Autodesk Inventor part; units mm, degrees
ref_plane "YZ Plane" through (0, 0, 0) normal (1, 0, 0) x (0, 1, 0)
ref_plane "XZ Plane" through (0, 0, 0) normal (0, 1, 0) x (-1, 0, 0)
ref_plane "XY Plane" through (0, 0, 0) normal (0, 0, 1) x (1, 0, 0)
sketch "Skizze2" plane through (0, 0, 0) normal (0, 1, 0) x (-1, 0, 0)
  line L0 (150, 125) -> (-150, 125)
  line L1 (-150, 125) -> (-150, -125)
  line L2 (-150, -125) -> (150, -125)
  line L3 (150, -125) -> (150, 125)
  point P0 (0, 0)
  dimension "d0" = 300
  dimension "d1" = 250
  dimension "d6" = 125
  dimension "d7" = 150
extrude "Extrusion1" add sketch "Skizze2" along normal blind 15
sketch "Skizze3" plane through (0, 15, 0) normal (0, 1, 0) x (1, 0, 0)
  circle A0 centre (0, -70.5) radius 3.25
  circle A1 centre (0, 70.5) radius 3.25
  point P0 (0, 0)
  dimension "d8" = 6.5
  dimension "d9" = 6.5
  dimension "d16" = 70.5
  dimension "d17" = 70.5
extrude "Extrusion2" cut sketch "Skizze3" against normal blind 15
sketch "Skizze4" plane through (0, 0, 0) normal (0, -1, 0) x (1, 0, 0)
  circle A0 centre (0, 70.5) radius 6.5
  circle A1 centre (0, -70.5) radius 6.5
  point P0 (0, 0)
  dimension "d12" = 13
  dimension "d13" = 13
  dimension "d18" = 70.5
  dimension "d19" = 70.5
extrude "Extrusion3" cut sketch "Skizze4" against normal blind 7
chamfer "Fase1" distance 2 angle 45 4 edges at (0, 15, 125) (150, 15, 0) (0, 15, -125) (-150, 15, 0)
sketch "Skizze5" plane through (0, 15, 0) normal (0, 1, 0) x (1, 0, 0)
  circle A0 centre (142.5, -42.5) radius 2.5
  circle A1 centre (97.5, -42.5) radius 2.5
  circle A2 centre (-142.5, 42.5) radius 2.5
  circle A3 centre (-97.5, 42.5) radius 2.5
  point P0 (0, 0)
  dimension "d23" = 5
  dimension "d24" = 5
  dimension "d25" = 5
  dimension "d26" = 5
extrude "Extrusion4" cut sketch "Skizze5" against normal blind 20
thread "Gewinde1"
thread "Gewinde2"
thread "Gewinde3"
thread "Gewinde4"
properties part number "Bodenplatte"
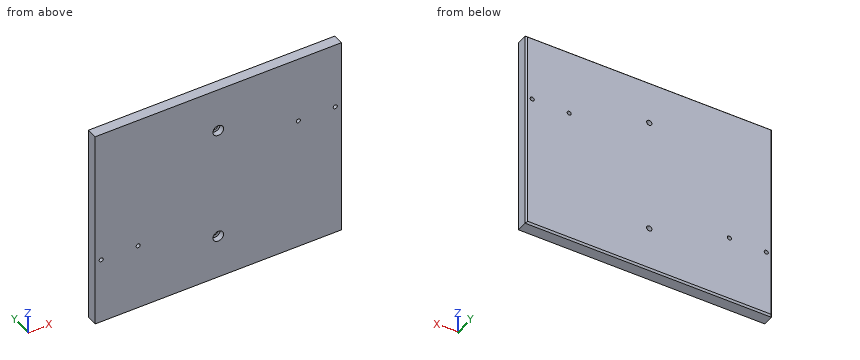
Could you check a few things on this model? Use its own coordinates, in mm. Coordinates: 2 decimals unless noted, no trailing zeros. Loops run counter-clockwise (first coordinate to the right, second up) from the corner with the lowest first, then second, coordinate; pieces in that order, holes last.
1. Imagine slicing it at A-A (x = 0). Please give me the cut outline in (y, z).
2. Imagine slicing it at B-B (z = 70.5). Please give me the cut outline in (x, y).
3. I need wall thicknesses on L1, parallel to X at y = 9.75, z = -42.5; L2, parallel to Z at x = 0, y = 5.25; L3, parallel to Z at x = 0, y = 10.25. Which ranges of each line are inside material? Lowest first, please.
4. For P1, Ø6.5, axis at x = 0.5, z = 69, coming from the -Y side, with a flat end and sliding along its axis, tell me the tip position at first contact or that it passes through.
Computed values:
1. outline: (0, -125) - (13, -125) - (15, -123) - (15, -73.75) - (7, -73.75) - (7, -77) - (0, -77) - close; (0, -64) - (7, -64) - (7, -67.25) - (15, -67.25) - (15, 67.25) - (7, 67.25) - (7, 64) - (0, 64) - close; (0, 77) - (7, 77) - (7, 73.75) - (15, 73.75) - (15, 123) - (13, 125) - (0, 125) - close
2. outline: (-150, 0) - (-6.5, 0) - (-6.5, 7) - (-3.25, 7) - (-3.25, 15) - (-148, 15) - (-150, 13) - close; (3.25, 7) - (6.5, 7) - (6.5, 0) - (150, 0) - (150, 13) - (148, 15) - (3.25, 15) - close
3. L1: x = -150 to -145, -140 to -100, -95 to 150
3. L2: z = -125 to -77, -64 to 64, 77 to 125
3. L3: z = -125 to -73.75, -67.25 to 67.25, 73.75 to 125
4. P1: stops at y = 7
